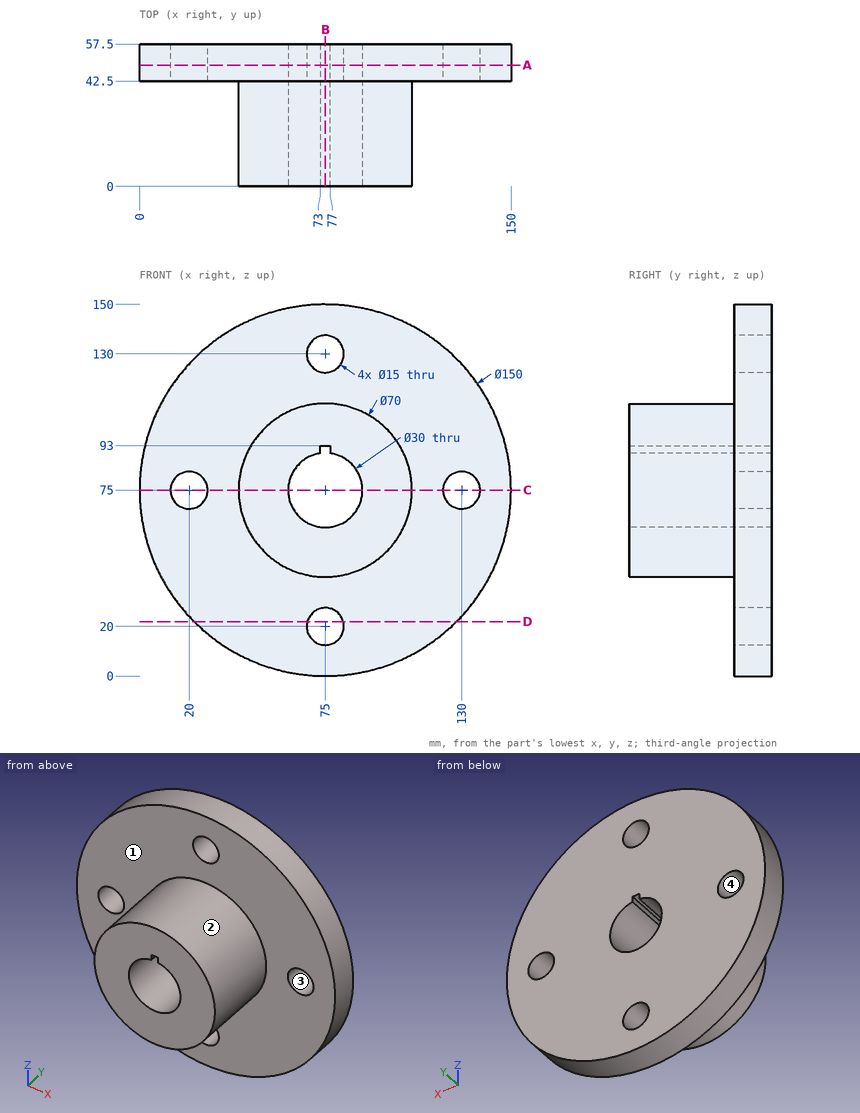
Check sheet for the drawn part. Datum: minimum x, y, z corner. Units: mm. Give positions to 0.01 mm unless a question says otherwise; leave off trailing zeros. Order: outer loops, then holes, each group sorted by start corner. A loop starts at its lowest first (then second) coordinate and runs counter-clockwise, first axis right, second up. Notation, with made-up numbers: (53.25, 32) - (58.25, 32) arc R15 cw to (58.25, 49) - close; hole circle Ø2 at (22.5, 82). An arc over 180 degrees is marked (long way). Answer in a Markdown table with one row per item. Add a question column.
Q1. Cross-section at A-A, the plane y = 49. Enter the section's corners in (x, z), then the cut area to 3 significant figures.
Q2. Gauge pin test, flat ends, axial feed: pin 1 (3 mm diameter, centred on x = 60, y = 21, fed in from -Z); pin 2 (1.5 mm diameter, centred on x = 53.5, y = 51.5, fed in from -Z); pin 3 (12 mm diameter, centred on x = 33.5, z = 30, fed in from -Y). Record the tip position at first contact, or that the pin passes through.
Q3. Material ranges on probe 1 along Z at (x, y) = (75, 49); probe 2 along Z at (x, y) = (75, 17); probe 3 along Y at (x, z) = (112, 104), recorded low to high. Write a range as from..to.
Q4. Cross-section at C-C, the plane z = 75. Enter the section's corners in (x, y).
Q5. Cross-section at B-B, the plane x = 75. Enter the section's corners in (y, z), then the cut area to 3 significant figures.
Q6. Mould release check, pull along X, two halves, no side actions. Record for the marked faces 1, 2, 3 and 4: pulls with the +X half, pulls with the -X half, needs draft (parallel to the pull), parting line crosses it, or undercut.
Q7. Cross-section at D-D, the plane z = 22. Enter the section's corners in (x, y).
Check values:
| question | item | result |
|---|---|---|
| 1 | outline | circle Ø150 at (75, 75); hole circle Ø15 at (20, 75); hole circle Ø15 at (75, 20); hole circle Ø15 at (75, 130); hole (73, 89.87) arc R15 ccw (long way) to (77, 89.87) - (77, 93) - (73, 93) - close; hole circle Ø15 at (130, 75) |
| 1 | area | 16,200 mm^2 |
| 2 | pin 1 | stops at z = 42.71 |
| 2 | pin 2 | stops at z = 2.93 |
| 2 | pin 3 | stops at y = 42.5 |
| 3 | probe 1 | z = 0..12.5, 27.5..60, 93..122.5, 137.5..150 |
| 3 | probe 2 | z = 40..60, 93..110 |
| 3 | probe 3 | y = 42.5..57.5 |
| 4 | outline | (0, 42.5) - (12.5, 42.5) - (12.5, 57.5) - (0, 57.5) - close; (27.5, 42.5) - (40, 42.5) - (40, 0) - (60, 0) - (60, 57.5) - (27.5, 57.5) - close; (90, 0) - (110, 0) - (110, 42.5) - (122.5, 42.5) - (122.5, 57.5) - (90, 57.5) - close; (137.5, 42.5) - (150, 42.5) - (150, 57.5) - (137.5, 57.5) - close |
| 5 | outline | (0, 40) - (42.5, 40) - (42.5, 27.5) - (57.5, 27.5) - (57.5, 60) - (0, 60) - close; (0, 93) - (57.5, 93) - (57.5, 122.5) - (42.5, 122.5) - (42.5, 110) - (0, 110) - close; (42.5, 0) - (57.5, 0) - (57.5, 12.5) - (42.5, 12.5) - close; (42.5, 137.5) - (57.5, 137.5) - (57.5, 150) - (42.5, 150) - close |
| 5 | area | 2,880 mm^2 |
| 6 | face 1 | needs draft |
| 6 | face 2 | parting line crosses it |
| 6 | face 3 | undercut |
| 6 | face 4 | undercut |
| 7 | outline | (21.93, 42.5) - (67.77, 42.5) - (67.77, 57.5) - (21.93, 57.5) - close; (82.23, 42.5) - (128.07, 42.5) - (128.07, 57.5) - (82.23, 57.5) - close |
